```python
from build123d import *

# Parameters (mm, degrees)
SKETCH1_R               = 3
BOSS_EXTRUDE1_DEPTH     = 12
CUT_EXTRUDE1_DEPTH      = 34.778691508
CUT_EXTRUDE1_DEPTH_BACK = 34.778691508
SKETCH3_R               = 6
SKETCH3_R_2             = 3
BOSS_EXTRUDE2_DEPTH     = 13


with BuildPart() as part:
    # Sketch1 → Boss-Extrude1 (new, symmetric)
    with BuildSketch(Plane.XY):
        with BuildLine():
            Line((0, -6), (-31, -6))
            Line((-31, -6), (-31, 6))
            Line((-31, 6), (0, 6))
            ThreePointArc((0, 6), (6, 0), (0, -6))
        make_face()
        Circle(SKETCH1_R, mode=Mode.SUBTRACT)
    extrude(amount=BOSS_EXTRUDE1_DEPTH, both=True)

    # Sketch2 → Cut-Extrude1 (cut, two sides: drawn at the far end of the back side and taken through both)
    with BuildSketch(Plane(origin=(0, 0, 0), x_dir=(1, 0, 0), z_dir=(0, 1, 0)).offset(-CUT_EXTRUDE1_DEPTH_BACK)):
        with BuildLine():
            Line((-15, 6), (6, 6))
            Line((6, 6), (6, -6))
            Line((6, -6), (-15, -6))
            ThreePointArc((-15, -6), (-21, 0), (-15, 6))
        make_face()
        Polygon((-31, 6), (-25, 12), (-31, 12), align=None)
        Polygon((-31, -12), (-31, -6), (-25, -12), align=None)
    extrude(amount=CUT_EXTRUDE1_DEPTH + CUT_EXTRUDE1_DEPTH_BACK, mode=Mode.SUBTRACT)

    # Sketch3 → Boss-Extrude2 (add)
    with BuildSketch(Plane.ZY.offset(31)):
        Circle(SKETCH3_R)
        with Locations(Location((0, 0, 0), (0, 0, 180))):
            Circle(SKETCH3_R_2, mode=Mode.SUBTRACT)
    extrude(amount=BOSS_EXTRUDE2_DEPTH)


solid = part.part
```
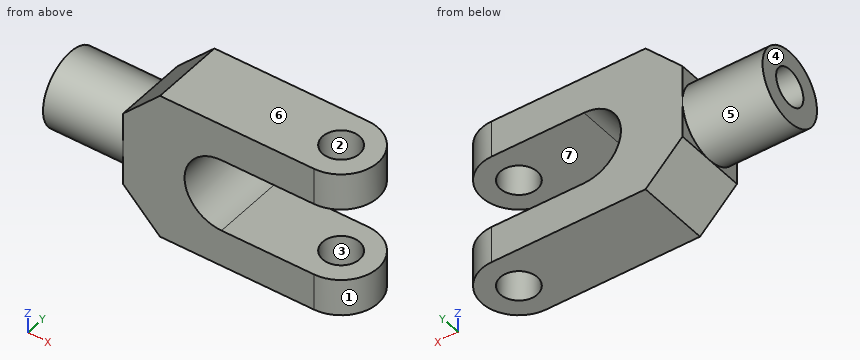
CAD build for the part. Positions are in the model's coordinates, mm. Face numbers are marked on the shaded views. A direction names the side the tool comes from. Round coordinates to 2 decimals unless told otherwise and drop trailing zeros. Order: outer loops, then holes, each group sorted by start corner. A loop starts at its lowest first (then second) coordinate and runs counter-clockwise, first axis right, second up.
Item 1: Tool access for the marked faces 5, 6 and 7: list every direction of +Z, -Z, +X, -X, +Y, -Y with a clear straight run to the whole face (end or side of a thin tool).
Item 2: Saw through at D-D on x = -37. Write the cut outline in (y, z).
Item 3: Pin check, flat tips, straight feed: pin 1 (3.5 mm diameter, centred on x = 0, y = 0, fed in from -Z); pin 2 (1 mm diameter, centred on y = 2, z = 0.5, fed in from +X); pin 3 (6 mm diameter, centred on y = 1.5, z = 1, fed in from +X). Stop position of each tip, or through.
Item 4: Saw through at C-C on y = 0.5. State how many separate pieces and enclosed holes the cut face has, then the cut area to 3 significant figures.
Item 5: Probe line 1 along Y through (x, z) = (0, -9.35); line 2 along Z through (x, y) = (-12, 1.75); line 3 along Z through (x, y) = (-39, -0.25). List the from-to ranges inside material, lowest first.
Item 6: Mould opens along X. For the marked faces 1, 2, 3 and 4 say: pulls with the +X half, pulls with the -X half, needs draft (parallel to the pull), parting line crosses it, or undercut.
Item 7: Saw through at B-B on z = -7.5. Write the cut outline in (x, y), then the cut area to 3 significant figures.
Item 8: Saw through at A-A on x = -13. Write the cut outline in (y, z), then the cut area to 3 significant figures.
Reported:
1. face 5: -X
1. face 6: +Z, +X, -X, +Y, -Y
1. face 7: +X, +Y, -Y
2. outline: circle Ø12 at (0, 0); hole circle Ø6 at (0, 0)
3. pin 1: passes through
3. pin 2: stops at x = -20.92
3. pin 3: stops at x = -19.47
4. separate pieces: 3
4. enclosed holes: 0
4. area: 551 mm2
5. line 1: y = -6 to -3, 3 to 6
5. line 2: z = -12 to -6, 6 to 12
5. line 3: z = -5.99 to -2.99, 2.99 to 5.99
6. face 1: pulls with the +X half
6. face 2: undercut
6. face 3: undercut
6. face 4: pulls with the -X half
7. outline: (-29.5, -6) - (0, -6) arc R6 ccw to (0, 6) - (-29.5, 6) - close; hole circle Ø6 at (0, 0)
7. area: 382 mm2
8. outline: (-6, -12) - (6, -12) - (6, -6) - (-6, -6) - close; (-6, 6) - (6, 6) - (6, 12) - (-6, 12) - close
8. area: 144 mm2
